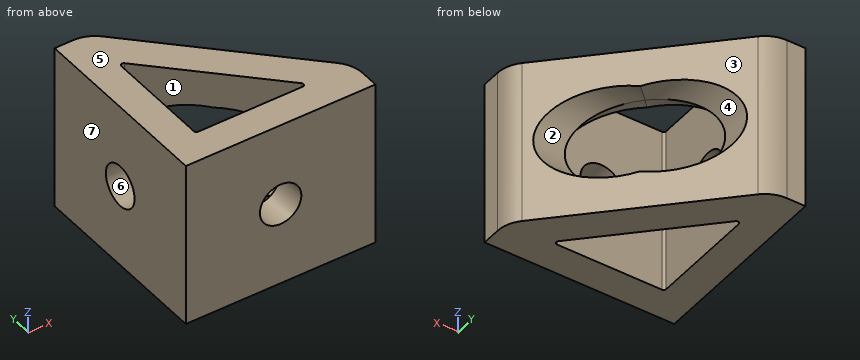
from build123d import *

# Parameters (mm, degrees)
BOSS_EXTRUDE2_DEPTH = 16.6624
CUT_EXTRUDE1_REACH  = 58.399
SKETCH3_R           = 4.16941
SKETCH4_R           = 9.525
CUT_EXTRUDE2_DEPTH  = 36.068
CUT_EXTRUDE3_REACH  = 58.399
SKETCH5_R           = 4.1656
SKETCH6_R           = 9.525
CUT_EXTRUDE4_DEPTH  = 36.068


with BuildPart() as part:
    # Sketch2 → Boss-Extrude2 (new, symmetric)
    with BuildSketch(Plane.XY):
        with BuildLine():
            Line((0, 38.1), (0, 0))
            Line((0, 0), (38.1, 0))
            Line((38.1, 0), (38.1, 3.719743879))
            ThreePointArc((38.1, 3.719743879), (37.616635031, 6.149783674), (36.240128061, 8.209871939))
            Line((36.240128061, 8.209871939), (8.209871939, 36.240128061))
            ThreePointArc((8.209871939, 36.240128061), (6.149783674, 37.616635031), (3.719743879, 38.1))
            Line((3.719743879, 38.1), (0, 38.1))
        make_face()
        with BuildLine():
            Line((6.35, 27.893323389), (6.35, 6.858))
            ThreePointArc((6.35, 6.858), (6.498789755, 6.498789755), (6.858, 6.35))
            Line((6.858, 6.35), (27.893323389, 6.35))
            ThreePointArc((27.893323389, 6.35), (28.362654192, 6.663596816), (28.252533634, 7.217210245))
            Line((28.252533634, 7.217210245), (7.217210245, 28.252533634))
            ThreePointArc((7.217210245, 28.252533634), (6.663596816, 28.362654192), (6.35, 27.893323389))
        make_face(mode=Mode.SUBTRACT)
    extrude(amount=BOSS_EXTRUDE2_DEPTH, both=True)

    # Sketch3 → Cut-Extrude1 (cut, up to next)
    with BuildSketch(Plane.ZY, mode=Mode.PRIVATE) as cut_extrude1_sk1:
        with Locations(Location((0, 19.05, 0), (0, 0, 270))):
            Circle(SKETCH3_R)
    cut_extrude1_tool1 = extrude(cut_extrude1_sk1.sketch, amount=-CUT_EXTRUDE1_REACH, mode=Mode.PRIVATE) & part.part
    add(cut_extrude1_tool1.solids().sort_by_distance((0, 19.05, 0))[0], mode=Mode.SUBTRACT)

    # Sketch4 → Cut-Extrude2 (cut)
    with BuildSketch(Plane(origin=(6.35, 0, 0), x_dir=(0, 0, -1), z_dir=(1, 0, 0))):
        with Locations(Location((0, 19.05, 0), (0, 0, 111.808163998))):
            Circle(SKETCH4_R)
    extrude(amount=CUT_EXTRUDE2_DEPTH, mode=Mode.SUBTRACT)

    # Sketch5 → Cut-Extrude3 (cut, up to next)
    with BuildSketch(Plane.XZ, mode=Mode.PRIVATE) as cut_extrude3_sk1:
        with Locations(Location((19.05, 0, 0), (0, 0, 270))):
            Circle(SKETCH5_R)
    cut_extrude3_tool1 = extrude(cut_extrude3_sk1.sketch, amount=-CUT_EXTRUDE3_REACH, mode=Mode.PRIVATE) & part.part
    add(cut_extrude3_tool1.solids().sort_by_distance((19.05, 0, 0))[0], mode=Mode.SUBTRACT)

    # Sketch6 → Cut-Extrude4 (cut)
    with BuildSketch(Plane(origin=(0, 6.35, 0), x_dir=(1, 0, 0), z_dir=(0, 1, 0))):
        with Locations((19.05, 0)):
            Circle(SKETCH6_R)
    extrude(amount=CUT_EXTRUDE4_DEPTH, mode=Mode.SUBTRACT)


solid = part.part
CAD build for the part. Positions are in the model's coordinates, mm. Face numbers are marked on the shaded views. A direction names the side the tool comes from. Coordinates: 2 decimals unless noted, no trailing zeros. Write each loop counter-clockwise with the first axis right and the second up, starting at its lowest first coordinate (ties: lowest second). Pieces come first, ordered by that corner, then holes. Notation, with made-up numbers: M 86.5,-25.5 L 90.5,-25.5 A32 cw 90.5,13.5 Z; hole C -36.75,84 d5. An arc over 180 degrees is marked long. Return JSON: item names as keys, results as strings.
Item 1: Slice it at A-A, the plane z = 0. Write the cut outline in (x, y) (3 decimals), and give its area (3 significant figures).
Findings below:
{"outline": "M 0,0 L 14.884,0 L 14.884,6.35 L 6.858,6.35 A0.508 cw 6.35,6.858 L 6.35,14.881 L 0,14.881 Z; M 0,23.219 L 6.35,23.219 L 6.35,28.575 L 9.525,28.575 L 9.525,34.925 L 8.21,36.24 A6.35 ccw 3.72,38.1 L 0,38.1 Z; M 23.216,0 L 38.1,0 L 38.1,3.72 A6.35 ccw 36.24,8.21 L 34.925,9.525 L 28.575,9.525 L 28.575,6.35 L 23.216,6.35 Z", "area": "386 mm2"}
Item 2: Drop flat-ended pins along their axis: pin 1 Ø6.5 at (y, z) = (13, -5) entering from +X; pin 2 Ø9.5 at (x, z) = (19.05, 0) entering from +Y; pin 3 Ø6.5 at (y, z) = (19.05, 0) entering from +X; pin 4 Ø11.5 at (y, z) = (19.05, 0) entering from +X. Give the stop position or say it passes through.
Findings below:
{"pin 1": "stops at x = 34.7", "pin 2": "stops at y = 6.35", "pin 3": "passes through", "pin 4": "stops at x = 6.35"}
Item 3: Slice it at C-C, the plane z = 10.5. Write the cut outline in (x, y).
Findings below:
{"outline": "M 0,0 L 38.1,0 L 38.1,3.72 A6.35 ccw 36.24,8.21 L 8.21,36.24 A6.35 ccw 3.72,38.1 L 0,38.1 Z; hole M 6.35,6.86 A0.51 ccw 6.86,6.35 L 27.89,6.35 A0.51 ccw 28.25,7.22 L 7.22,28.25 A0.51 ccw 6.35,27.89 Z"}
Item 4: Slice it at B-B, the plane y = 16. Write the cut outline in (x, z) (3 decimals).
Findings below:
{"outline": "M 0,-16.662 L 6.35,-16.662 L 6.35,-2.843 L 0,-2.843 Z; M 0,2.843 L 6.35,2.843 L 6.35,16.662 L 0,16.662 Z; M 19.47,-16.662 L 28.45,-16.662 L 28.45,-9.023 L 22.1,-9.023 A9.525 cw 19.47,-9.516 Z; M 19.47,9.516 A9.525 cw 22.1,9.023 L 28.45,9.023 L 28.45,16.662 L 19.47,16.662 Z"}
Item 5: Two-plate mould, pull along Z, no slides. Class the marked faces 5, 6 and 7: +Z half, -Z half, draft (parallel to the pull), parting line (faces both ways), or undercut.
Findings below:
{"face 5": "+Z half", "face 6": "undercut", "face 7": "draft"}
Item 6: Which spindle directions (+Z, -Z, +X, -X, +Y, -Y) get a long thin tool onto all of the face, cutting with end or side? Do the marked faces 1, 2, 3 and 4. Say none if no direction does.
Findings below:
{"face 1": "+Z, -Z", "face 2": "+X", "face 3": "+Z, -Z, +X, +Y", "face 4": "+Y"}
Item 7: Slice it at D-D, the plane x = 17. Write the cut outline in (y, z) (3 decimals).
Findings below:
{"outline": "M 0,-16.662 L 6.35,-16.662 L 6.35,-3.626 L 0,-3.626 Z; M 0,3.626 L 6.35,3.626 L 6.35,16.662 L 0,16.662 Z; M 18.47,-16.662 L 27.45,-16.662 L 27.45,-9.302 L 21.1,-9.302 A9.525 cw 18.47,-9.507 Z; M 18.47,9.507 A9.525 cw 21.1,9.302 L 27.45,9.302 L 27.45,16.662 L 18.47,16.662 Z"}
Item 8: Probe line 1 (Z direction, x = 4, y = 19.05); line 2 (X direction, y = 4, z = 0); line 3 (Y direction, x = 15.5, z = 2.5). List the from-to ranges inside material, lowest first. Write a range as from..to.
Findings below:
{"line 1": "z = -16.66..-4.17, 4.17..16.66", "line 2": "x = 0..14.88, 23.22..38.09", "line 3": "y = 0..6.35"}
